Can you work these out from the model? Positions are in its coordinate system, mm. Face numbers are marked on the shaded views. A direction names the side the tool comes from. Round coordinates to 2 decimals unless told otherwise and drop trailing zeros. Loops run counter-clockwise (first coordinate to the right, second up) from the corner with the lowest first, then second, coordinate; pieces in that order, holes last.
from build123d import *

# Parameters (mm, degrees)
BOSS_EXTRUDE1_DEPTH                      = 50
CBORE_FOR_M5_PAN_HEAD_SCREW1_D           = 5.5
CBORE_FOR_M5_PAN_HEAD_SCREW1_DEPTH       = 30
CBORE_FOR_M5_PAN_HEAD_SCREW1_CBORE_D     = 11
CBORE_FOR_M5_PAN_HEAD_SCREW1_CBORE_DEPTH = 3.7
CBORE_FOR_M5_PAN_HEAD_SCREW1_TIP         = 1.652366702


with BuildPart() as part:
    # Sketch2 → Boss-Extrude1 (new body)
    with BuildSketch(Plane(origin=(0, 0, 0), x_dir=(0, 0, -1), z_dir=(1, 0, 0))):
        with BuildLine():
            Line((0, 0), (0, 70))
            Line((0, 70), (5, 70))
            Line((5, 70), (5, 15))
            ThreePointArc((5, 15), (7.928932188, 7.928932188), (15, 5))
            Line((15, 5), (35, 5))
            Line((35, 5), (35, 0))
            Line((35, 0), (0, 0))
        make_face()
    extrude(amount=BOSS_EXTRUDE1_DEPTH)

    # CBORE for M5 Pan Head Screw1
    with Locations(Plane(origin=(0, 5, 0), x_dir=(1, 0, 0), z_dir=(0, 1, 0))):
        with Locations((40, 25), (10, 25)):
            CounterBoreHole(CBORE_FOR_M5_PAN_HEAD_SCREW1_D / 2, CBORE_FOR_M5_PAN_HEAD_SCREW1_CBORE_D / 2, CBORE_FOR_M5_PAN_HEAD_SCREW1_CBORE_DEPTH, depth=CBORE_FOR_M5_PAN_HEAD_SCREW1_DEPTH)
            with Locations((0, 0, -(CBORE_FOR_M5_PAN_HEAD_SCREW1_DEPTH + CBORE_FOR_M5_PAN_HEAD_SCREW1_TIP / 2))):  # 118° drill point
                Cone(0, CBORE_FOR_M5_PAN_HEAD_SCREW1_D / 2, CBORE_FOR_M5_PAN_HEAD_SCREW1_TIP, mode=Mode.SUBTRACT)


solid = part.part
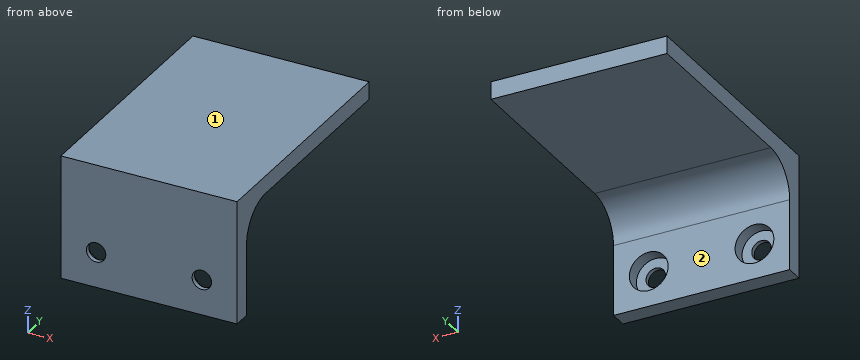
(1) If we section it at D-D, the plane x = 41.5: List the corners of the cut face in (y, z) for me, then the cut area to 3 significant figures.
Worked answers:
outline: (0, -35) - (5, -35) - (5, -30.29) - (1.3, -30.29) - (1.3, -27.3) - (0, -27.3) - close; (0, -22.7) - (1.3, -22.7) - (1.3, -19.71) - (5, -19.71) - (5, -15) arc R10 cw to (15, -5) - (70, -5) - (70, 0) - (0, 0) - close
area: 476 mm2
(2) If we section it at C-C, the plane y = 37.5: List the corners of the cut face in (x, z) for me.
Worked answers:
outline: (0, -5) - (50, -5) - (50, 0) - (0, 0) - close
(3) For the marked faces 1 and 2, which set-ups out of +Z, -Z, +X, -X, +Y, -Y let a thin tool reach every point of the face, with its end or its side?
Worked answers:
face 1: +Z, +X, -X, +Y, -Y
face 2: -Z, +X, -X, +Y
(4) If I drill on line 1 (X direction, y = 0.3, z = -25); line 2 (X direction, y = 3.85, z = -25); line 3 (Z direction, x = 40, y = 4.05), over which ranges is the centre line in solid material (lowest first)?
Worked answers:
line 1: x = 0 to 7.25, 12.75 to 37.25, 42.75 to 50
line 2: x = 0 to 4.5, 15.5 to 34.5, 45.5 to 50
line 3: z = -35 to -30.5, -19.5 to 0
(5) Will these pins go through, and if not, where does the flat tip stop? P1, Ø12.5, axis at x = 40, z = -25, coming from the -Y side; P2, Ø1, axis at x = 20, z = -11, coming from the +Y side; P3, Ø6, axis at x = 14.5, z = -30, coming from the +Y side; P4, Ø3.5, axis at x = 38, z = -24, coming from the +Y side.
Worked answers:
P1: stops at y = 0
P2: stops at y = 6.07
P3: stops at y = 5
P4: stops at y = 1.3
(6) If we section it at B-B, the plane z = -25: List the corners of the cut face in (x, y) for me, then the cut area to 3 significant figures.
Worked answers:
outline: (0, 0) - (7.25, 0) - (7.25, 1.3) - (4.5, 1.3) - (4.5, 5) - (0, 5) - close; (12.75, 0) - (37.25, 0) - (37.25, 1.3) - (34.5, 1.3) - (34.5, 5) - (15.5, 5) - (15.5, 1.3) - (12.75, 1.3) - close; (42.75, 0) - (50, 0) - (50, 5) - (45.5, 5) - (45.5, 1.3) - (42.75, 1.3) - close
area: 154 mm2
(7) If we section it at A-A, the plane x = 10: List the corners of the cut face in (y, z) for me.
Worked answers:
outline: (0, -35) - (5, -35) - (5, -30.5) - (1.3, -30.5) - (1.3, -27.75) - (0, -27.75) - close; (0, -22.25) - (1.3, -22.25) - (1.3, -19.5) - (5, -19.5) - (5, -15) arc R10 cw to (15, -5) - (70, -5) - (70, 0) - (0, 0) - close
